Part model, mm, in its own coordinate system. A direction names the side the tool comes from. Round coordinates to 2 decimals unless told otherwise and drop trailing zeros. Write each question's results on one line, items separated by ' | '. Start each with the question number.
1. Drop flat-ended pins along their axis: pin 1 Ø3.5 at (x, y) = (33.38, 8.94) entering from +Z; pin 2 Ø5 at (x, y) = (19, 6.5) entering from +Z; pin 3 Ø6 at (x, z) = (15, 36) entering from +Y; pin 4 Ø6 at (x, y) = (20.5, 31.5) entering from +Z. Give the stop position or say it passes through.
2. Two-plate mould, pull along X, no slides. Class faces 1 (the face through (6, 6, 41)), 2 (the face through (15.648, 15.328, 21.905)), 3 (the face through (7.92, 34.98, 0.34)): +X half, -X half, draft (parallel to the pull), parting line (faces both ways), or undercut.
3. Which spindle directions (+Z, -Z, +X, -X, +Y, -Y) get a long thin tool onto all of the face, cutting with end or side? Do faces 4 (the face through (31.568, 9.514, 0.345)), 5 (the face through (23, 23, 3)). Say none if no direction does.
4. Probe L1, parallel to Z at x = 32, y = 21.5; L2, parallel to Y at x = 4.5, z = 4.5; L3, parallel to Z at x = 35.5, y = 20. List the from-to ranges inside material, lowest first. Write a range as [from, to].
```python
from build123d import *

# Parameters (mm, degrees)
F1_ANGLE       = 90
F3_D           = 3.7973
F3_CSINK_D     = 7.7978
F3_CSINK_ANGLE = 82
F4_R           = 1


with BuildPart() as f1:
    # F0 (on Front) → F1 (revolve)
    with BuildSketch(Plane.XZ):
        with BuildLine():
            ThreePointArc((29.5563491861, 3), (19.3936743285, 9.790482244), (21.7781745931, 21.7781745931))
            Line((21.7781745931, 21.7781745931), (22.2218254069, 22.2218254069))
            ThreePointArc((22.2218254069, 22.2218254069), (24.6063256715, 34.209517756), (14.4436508139, 41))
            Line((14.4436508139, 41), (0, 41))
            Line((0, 41), (0, 0))
            Line((0, 0), (39.5563491861, 0))
            ThreePointArc((39.5563491861, 0), (41.0563491861, 1.5), (39.5563491861, 3))
            Line((39.5563491861, 3), (29.5563491861, 3))
        make_face()
    revolve(axis=Axis((0, 0, 20.5), (0, 0, 1)), revolution_arc=F1_ANGLE)

    # F3 (through all)
    with Locations(Plane.XY.offset(3)):
        with Locations((8.9438412986, 33.3788701411), (33.3788701411, 8.9438412986)):
            CounterSinkHole(F3_D / 2, F3_CSINK_D / 2, counter_sink_angle=F3_CSINK_ANGLE)

    # F4
    f4_edges = [f1.edges().sort_by_distance(p)[0] for p in [
        (19.393674, 0, 9.790482),
        (22, 0, 22),
        (24.606326, 0, 34.209518),
        (7.221825, 0, 41),
        (0, 0, 20.5),
        (19.778175, 0, 0),
        (41.056349, 0, 1.5),
        (34.556349, 0, 3),
        (0, 19.393674, 9.790482),
        (0, 22, 22),
        (0, 24.606326, 34.209518),
        (0, 7.221825, 41),
        (0, 19.778175, 0),
        (0, 41.056349, 1.5),
        (0, 34.556349, 3),
    ]]
    fillet(f4_edges, radius=F4_R)


solid = f1.part
```
Solution:
1) pin 1: through | pin 2: z = 40.54 | pin 3: y = 21.14 | pin 4: z = 3
2) face 1: draft | face 2: +X half | face 3: undercut
3) face 4: +Z, -Z | face 5: +Z, +X, +Y
4) L1: [0, 3] | L2: [0, 23.59] | L3: [0.59, 2.41]
